```python
from build123d import *

# Parameters (mm, degrees)
CROQUIS1_R              = 7.5
CROQUIS1_R_2            = 3.5
SALIENTE_EXTRUIR1_DEPTH = 4
CROQUIS2_R              = 2.193779366
SALIENTE_EXTRUIR2_DEPTH = 5
CROQUIS3_R              = 7.5
CROQUIS3_R_2            = 3.5
SALIENTE_EXTRUIR3_DEPTH = 4
CROQUIS4_R              = 2.193779366
CORTAR_EXTRUIR1_DEPTH   = 14
SALIENTE_EXTRUIR4_DEPTH = 13


with BuildPart() as part:
    # Croquis1 → Saliente-Extruir1 (new body)
    with BuildSketch(Plane.XY):
        Circle(CROQUIS1_R)
        Circle(CROQUIS1_R_2, mode=Mode.SUBTRACT)
    extrude(amount=SALIENTE_EXTRUIR1_DEPTH)



with BuildPart() as body_2:
    # Croquis2 → Saliente-Extruir2 (new body)
    with BuildSketch(Plane(origin=(0, 0, 0), x_dir=(-1, 0, 0), z_dir=(0, 0, -1))):
        Circle(CROQUIS2_R)
    extrude(amount=SALIENTE_EXTRUIR2_DEPTH)

    # Croquis4 → Cortar-Extruir1 (cut)
    with BuildSketch(Plane(origin=(0, 0, -5), x_dir=(-1, 0, 0), z_dir=(0, 0, -1))):
        Circle(CROQUIS4_R)
    extrude(amount=-CORTAR_EXTRUIR1_DEPTH, mode=Mode.SUBTRACT)


with BuildPart() as body_3:
    # Croquis3 → Saliente-Extruir3 (new body)
    with BuildSketch(Plane(origin=(0, 0, -5), x_dir=(-1, 0, 0), z_dir=(0, 0, -1))):
        Circle(CROQUIS3_R)
        Circle(CROQUIS3_R_2, mode=Mode.SUBTRACT)
    extrude(amount=SALIENTE_EXTRUIR3_DEPTH)


with BuildPart() as part_1:
    add(part.part)

    add(body_3.part)  # Saliente-Extruir4 merges body 3
    # Croquis5 → Saliente-Extruir4 (add)
    with BuildSketch(Plane.XY.offset(4)):
        with BuildLine():
            Line((-10.009282788, -8.566914266), (0, -7.5))
            ThreePointArc((0, -7.5), (-5.895156044, -4.636500319), (-7.288771435, 1.76743061))
            ThreePointArc((-7.288771435, 1.76743061), (-27.875344012, -0.49038836), (-46.981845806, 7.5))
            Line((-46.981845806, 7.5), (-46.981845806, 4.90393409))
            ThreePointArc((-46.981845806, 4.90393409), (-30.939741801, -8.539865418), (-10.009282788, -8.566914266))
        make_face()
    extrude(amount=-SALIENTE_EXTRUIR4_DEPTH)


solid = part_1.part
```
The model under review builds one solid part; all positions refer to its coordinate system, in mm. Coordinates: 2 decimals unless noted, no trailing zeros. Write each loop counter-clockwise with the first axis right and the second up, starting at its lowest first coordinate (ties: lowest second). Pieces come first, ordered by that corner, then holes. Notation, with made-up numbers: (-16.5, 30.25) -> (38.5, 30.25) arc R36 ccw to (38.5, 64.25) -> close; hole circle Ø7 at (-24, -23). An arc over 180 degrees is marked (long way). One line per item, written item: value. Start each with the question number.
Q1. To check wall thickness, follow probe 1 along Z at (x, y) = (4, 2.5); probe 2 along Y at (x, z) = (0, 1.8); probe 3 along X at (y, z) = (5.25, 1.5). State the ranges of each line that lie inside material, in increasing order.
Q2. Clearance check with flat-ended pins moving along their axes: P1, Ø6, axis at y = -4.5, z = -2.5, coming from the +X side; P2, Ø3, axis at x = -26.5, z = -4, coming from the -Y side. State where each tip first meets the part, or that it passes through.
Q3. Add section A-A, the plane y = 5.5. Give the boundary of the cut face in (x, z), then the cut area to 3 significant figures.
Q4. Add section B-B, the plane z = 1. Give the boundary of the cut face in (x, y), then the cut area to 3 significant figures.
Q5. The part is to be moulded in two halves that separate along Y. For faces 1 (the face through (-5.836, -4.711, -2.465)), 2 (the face through (-46.982, 6, -2)), 3 (the face through (5.747, 4.819, -6.972)), say which applies: +Y half, -Y half, draft (parallel to the pull), parting line (faces both ways), or undercut.
Q6. Add section C-C, the plane x = 1.5. Give the boundary of the cut face in (y, z).
Q7. Add section D-D, the plane y = 0. Give the boundary of the cut face in (x, z).
Response:
1. probe 1: -9 to -5, 0 to 4
1. probe 2: -7.5 to -3.5, 3.5 to 7.5
1. probe 3: -46.98 to -43.7, -5.36 to 5.36
2. P1: x = 6.94
2. P2: y = -10.05
3. outline: (-46.98, -9) -> (-44.1, -9) -> (-44.1, 4) -> (-46.98, 4) -> close; (-5.1, -9) -> (5.1, -9) -> (5.1, -5) -> (-5.1, -5) -> close; (-5.1, 0) -> (5.1, 0) -> (5.1, 4) -> (-5.1, 4) -> close
3. area: 119 mm²
4. outline: (-46.98, 4.9) arc R30.68 ccw to (-10.01, -8.57) -> (0, -7.5) arc R7.5 ccw (long way) to (-7.29, 1.77) arc R41.42 cw to (-46.98, 7.5) -> close; hole circle Ø7 at (0, 0)
4. area: 478 mm²
5. face 1: undercut
5. face 2: draft
5. face 3: parting line
6. outline: (-7.35, -9) -> (-3.16, -9) -> (-3.16, -5) -> (-7.35, -5) -> close; (-7.35, 0) -> (-3.16, 0) -> (-3.16, 4) -> (-7.35, 4) -> close; (3.16, -9) -> (7.35, -9) -> (7.35, -5) -> (3.16, -5) -> close; (3.16, 0) -> (7.35, 0) -> (7.35, 4) -> (3.16, 4) -> close
7. outline: (-43.45, -9) -> (-30.62, -9) -> (-30.62, 4) -> (-43.45, 4) -> close; (-13.29, -9) -> (-3.5, -9) -> (-3.5, -5) -> (-7.5, -5) -> (-7.5, 0) -> (-3.5, 0) -> (-3.5, 4) -> (-13.29, 4) -> close; (3.5, -9) -> (7.5, -9) -> (7.5, -5) -> (3.5, -5) -> close; (3.5, 0) -> (7.5, 0) -> (7.5, 4) -> (3.5, 4) -> close
